Model file for the job. Use its own axes, mm. A direction names the side the tool comes from. Round coordinates to 2 decimals unless told otherwise and drop trailing zeros. Order: outer loops, then holes, each group sorted by start corner. A loop starts at its lowest first (then second) coordinate and runs counter-clockwise, first axis right, second up. Notation, with made-up numbers: (69, 66) -> (79, 66) arc R22 cw to (79, 102) -> close; hole circle Ø8 at (41.25, 81.25). An arc over 180 degrees is marked (long way). Put each result on its own line as item: value. Start each with the question number.
Q1. Cut at A-A, the plane x = 39. List the corners of the cut face in (y, z) (1 decimal).
Q2. Probe L1, parallel to X at y = -0.5, z = 9; L2, parallel to Y at x = 6.5, z = 0; L3, parallel to X at y = -7.5, z = 12. List the from-to ranges inside material, lowest first.
Q3. Cut at B-B, the plane x = 19. List the corners of the cut face in (y, z).
Q4. 3-axis set-ups, long thin cutter, end or side, ignore diameter. For faces 1 (the face through (11.845, -1.061, -8.084)), 2 (the face through (-10.47, -6.99, -12.04)): which of +Z, -Z, +X, -X, +Y, -Y reach the whole face in a straight line?
Q5. Flat gauge pins, fed straight in: P1, Ø8, axis at x = 47, z = 0.5, coming from the -Y side; P2, Ø12, axis at x = 11.5, y = -2.5, coming from the -Z side; P3, Ø3, axis at x = 24.5, y = 0.5, coming from the +Z side. Where does each tip first touch, or does it go through?
Autodesk Inventor part; units mm, degrees
ref_plane "YZ Plane" through (0, 0, 0) normal (1, 0, 0) x (0, 1, 0)
ref_plane "XZ Plane" through (0, 0, 0) normal (0, 1, 0) x (-1, 0, 0)
ref_plane "XY Plane" through (0, 0, 0) normal (0, 0, 1) x (1, 0, 0)
sketch "Sketch1" plane through (0, 0, 0) normal (0, 0, 1) x (1, 0, 0)
  line L0 (0, 8.1534) -> (0, 8.1534)
  line L1 (25.4, 7.9375) -> (63.5, 7.9375)
  line L2 (63.5, 7.9375) -> (63.5, 0)
  line L3 (63.5, 0) -> (-0.0001, 0)
  line L4 (-6.3501, 0) -> (82.55, 0)
  line L5 (-0.0001, 0) -> (-0.0001, 8.1534)
  line L6 (-0.0001, 8.1534) -> (0, 8.1534)
  line L7 (25.4, 7.9375) -> (24.0258, 8.1534)
  line L8 (24.0258, 8.1534) -> (0, 8.1534)
  line L9 (0, -0.8153) -> (0, 10.5994)
  dimension "d0" = 63.5
  dimension "d1" = 38.1
  dimension "d2" = 15.875
  dimension "d9" = 0.0001
  dimension "d10" = 16.3068
  dimension "d13" = 1.3742
  dimension "d14" = 16.3068
revolve "Body" add sketch "Sketch1" angle 360 about axis through (63.5, 0, 0) along (-1, 0, 0)
sketch "Sketch2" plane through (-0.0001, 0, 0) normal (-1, 0, 0) x (0, 0, 1)
  line L0 (0, 15.5812) -> (13.4937, 7.7906)
  line L1 (13.4937, 7.7906) -> (13.4937, -7.7906)
  line L2 (13.4937, -7.7906) -> (0, -15.5812)
  line L3 (0, -15.5812) -> (-13.4937, -7.7906)
  line L4 (-13.4937, -7.7906) -> (-13.4937, 7.7906)
  line L5 (-13.4937, 7.7906) -> (0, 15.5812)
  point P0 (0, 0)
  point P1 (0, 0)
  dimension "d11" = 26.9875
extrude "Head" add sketch "Sketch2" along normal blind 10.7156
sketch "Sketch4" plane through (0, 0, 0) normal (0, 0, 1) x (1, 0, 0)
  line L0 (-10.7157, 13.4938) -> (-10.7157, 15.5812)
  line L1 (-10.7157, 15.5812) -> (-9.5105, 15.5812)
  line L2 (-9.5105, 15.5812) -> (-10.7157, 13.4938)
  line L3 (-11.7873, 0) -> (3.2146, 0)
  line L4 (-0.0001, 15.5812) -> (-10.7157, 15.5812)
  line L5 (-10.7157, 7.7906) -> (-10.7157, 15.5812)
  dimension "d5" = 30
  dimension "d19" = 26.9875
revolve "Chamfer1" cut sketch "Sketch4" angle 360 about axis through (-10, 0, 0) along (1, 0, 0)
thread "Thread"
chamfer "Chamfer2" distance 1.3741 distance2 1.3742 1 edges at (63.5, -7.9375, 0) measured on face at (63.5, -0.6813, 3.1515)
equation "\"d0\" = NLG"
equation "\"d1\" = GEL"
equation "\"d2\" = GD"
equation "\"d10\" = SD2"
equation "\"d14\" = BDM"
equation "\"d11\" = SW"
equation "\"d3\" = KOH - SD"
equation "\"d5\" = ANG1"
equation "\"d19\" = SW0"
equation "\"d15\" = GEL"
equation "\"d6\" = -0.5 * SPD + 0.5 * GD"
equation "\"NLG\" = 63.5"
equation "\"GD\" = NND"
equation "\"BDM\" = 16.3068"
equation "\"KOH\" = 10.71562"
equation "\"GEL\" = 38.1"
equation "\"SW\" = 26.9875"
equation "\"SW0\" = SW"
equation "\"SPD\" = 13.12672"
equation "\"SD2\" = BDM"
equation "\"SD\" = 0"
equation "\"ANG1\" = 30deg"
equation "\"GAL\" = GUL"
equation "\"GUL\" = 1.37414"
equation "\"RR\" = 1.524"
equation "\"d20\" = -NLG"
equation "\"TOA\" = 30deg"
equation "\"THREADDIA\" = 15.875"
equation "\"E0\" = 1.155 * SW"
equation "\"GD1\" = SPD"
equation "\"SLG\" = 19.62734"
equation "\"NND\" = 15.875"
properties part number "ANSI B18.2.1 - 5/8-11 UNC - 2.5"
Ans:
1. outline: circle Ø15.9 at (0, 0)
2. L1: x = -10.72 to 0
2. L2: y = -8.15 to 8.15
2. L3: x = -10.34 to 0
3. outline: circle Ø16.31 at (0, 0)
4. face 1: +X
4. face 2: -Z, -X, -Y
5. P1: stops at y = -7.94
5. P2: stops at z = -8.15
5. P3: stops at z = 8.15
